Can you work these out from the model? Positions are in its coordinate system, mm. A direction names the side the tool comes from. Coordinates: 2 decimals unless noted, no trailing zeros. Write each loop counter-clockwise with the first axis right and the second up, starting at its lowest first coordinate (ties: lowest second). Pieces come first, ordered by that corner, then holes.
```python
from build123d import *

# Parameters (mm, degrees)
BOSS_EXTRUDE1_DEPTH  = 5
SKETCH8_W            = 12.7
SKETCH8_H            = 25.4
CUT_EXTRUDE1_DEPTH   = 12.7
BOSS_EXTRUDE6_START  = 1.27
BOSS_EXTRUDE6_DEPTH  = 22.86
FILLET3_R            = 2.54
SKETCH12_W           = 22.86
SKETCH12_H           = 5.08
BOSS_EXTRUDE7_DEPTH  = 5.08
FILLET8_R            = 2.54
SKETCH13_W           = 2.54
SKETCH13_H           = 17.78
CUT_EXTRUDE2_DEPTH   = 2.032
BOSS_EXTRUDE8_DEPTH  = 22.86
FILLET5_R            = 2.54
FILLET6_R            = 2.54
BOSS_EXTRUDE9_START  = -27.94
SKETCH15_W           = 10.16
SKETCH15_H           = 3.81
BOSS_EXTRUDE9_DEPTH  = 12.7
BOSS_EXTRUDE10_START = -116.84
SKETCH15_2_W         = 10.16
SKETCH15_2_H         = 3.81
BOSS_EXTRUDE10_DEPTH = 12.7
FILLET7_R            = 2.54


with BuildPart() as part:
    # Sketch2 → Boss-Extrude1 (new body)
    with BuildSketch(Plane(origin=(0, 0, 0), x_dir=(1, 0, 0), z_dir=(0, 1, 0))):
        with BuildLine():
            Line((-98.109845206, -87.510053172), (49.730154794, -87.510053172))
            ThreePointArc((49.730154794, -87.510053172), (53.322257243, -86.02215562), (54.810154794, -82.430053172))
            Line((54.810154794, -82.430053172), (54.810154794, 64.409946828))
            ThreePointArc((54.810154794, 64.409946828), (53.322257243, 68.002049277), (49.730154794, 69.489946828))
            Line((49.730154794, 69.489946828), (-98.109845206, 69.489946828))
            ThreePointArc((-98.109845206, 69.489946828), (-101.701947654, 68.002049277), (-103.189845206, 64.409946828))
            Line((-103.189845206, 64.409946828), (-103.189845206, -82.430053172))
            ThreePointArc((-103.189845206, -82.430053172), (-101.701947654, -86.02215562), (-98.109845206, -87.510053172))
        make_face()
    extrude(amount=BOSS_EXTRUDE1_DEPTH)

    # Sketch8 → Cut-Extrude1 (cut)
    with BuildSketch(Plane(origin=(0, 5, 0), x_dir=(1, 0, 0), z_dir=(0, 1, 0))):
        with Locations((-96.839845206, -9.250053172)):
            Rectangle(SKETCH8_W, SKETCH8_H)
    extrude(amount=-CUT_EXTRUDE1_DEPTH, mode=Mode.SUBTRACT)

    # Sketch9 → Boss-Extrude6 (add)
    with BuildSketch(Plane(origin=(0, 0, 21.950053172), x_dir=(-1, 0, 0), z_dir=(0, 0, -1)).offset(BOSS_EXTRUDE6_START)):
        with BuildLine():
            Line((90.489845206, 5), (90.489845206, -9.510091846))
            ThreePointArc((90.489845206, -9.510091846), (91.233793982, -11.30614307), (93.029845206, -12.050091846))
            Line((93.029845206, -12.050091846), (100.984663509, -12.050091846))
            ThreePointArc((100.984663509, -12.050091846), (102.780714734, -11.30614307), (103.524663509, -9.510091846))
            Line((103.524663509, -9.510091846), (103.524663509, 5))
            Line((103.524663509, 5), (100.984663509, 5))
            Line((100.984663509, 5), (100.984663509, -6.970091846))
            ThreePointArc((100.984663509, -6.970091846), (100.240714734, -8.76614307), (98.444663509, -9.510091846))
            Line((98.444663509, -9.510091846), (97.007254358, -9.510091846))
            add(Edge.make_bspline(
                [(93.029845206, -3.470974905), (93.181288834, -7.756398779), (97.007254358, -9.510091846)],
                knots=[0, 0, 0, 1, 1, 1], degree=2))
            Line((93.029845206, -3.470974905), (93.029845206, 5))
            Line((93.029845206, 5), (90.489845206, 5))
        make_face()
    extrude(amount=BOSS_EXTRUDE6_DEPTH)

    # Fillet3
    fillet3_edges = [part.edges().sort_by_distance(p)[0] for p in [
        (-90.489845206, 0, 9.250053172),
    ]]
    fillet(fillet3_edges, radius=FILLET3_R)

    # Sketch12 → Boss-Extrude7 (add)
    with BuildSketch(Plane.ZY.offset(103.524663509)):
        with Locations((9.250053172, 2.46)):
            Rectangle(SKETCH12_W, SKETCH12_H)
    extrude(amount=BOSS_EXTRUDE7_DEPTH)

    # Fillet8
    fillet8_edges = [part.edges().sort_by_distance(p)[0] for p in [
        (-100.984663509, 5, 9.250053172),
    ]]
    fillet(fillet8_edges, radius=FILLET8_R)

    # Sketch13 → Cut-Extrude2 (cut)
    with BuildSketch(Plane(origin=(0, 5, 0), x_dir=(1, 0, 0), z_dir=(0, 1, 0))):
        with Locations((-106.064663509, -9.250053172)):
            Rectangle(SKETCH13_W, SKETCH13_H)
    extrude(amount=-CUT_EXTRUDE2_DEPTH, mode=Mode.SUBTRACT)

    # Sketch14 → Boss-Extrude8 (add)
    with BuildSketch(Plane(origin=(0, 0, -2.179946828), x_dir=(-1, 0, 0), z_dir=(0, 0, -1))):
        Polygon((103.524663509, -4.576775108), (105.048663509, -4.576775108), (103.524663509, -7.370775108), align=None)
    extrude(amount=-BOSS_EXTRUDE8_DEPTH)

    # Fillet5
    fillet5_edges = [part.edges().sort_by_distance(p)[0] for p in [
        (-93.029845206, 5, 9.250053172),
    ]]
    fillet(fillet5_edges, radius=FILLET5_R)

    # Fillet6
    fillet6_edges = [part.edges().sort_by_distance(p)[0] for p in [
        (-108.604663509, -0.08, 9.250053172),
    ]]
    fillet(fillet6_edges, radius=FILLET6_R)

    # Sketch15 → Boss-Extrude9 (add)
    with BuildSketch(Plane(origin=(0, 0, -69.489946828), x_dir=(-1, 0, 0), z_dir=(0, 0, -1)).offset(BOSS_EXTRUDE9_START)):
        with Locations((-54.290154794, -1.905)):
            Rectangle(SKETCH15_W, SKETCH15_H)
    extrude(amount=-BOSS_EXTRUDE9_DEPTH)

    # Sketch15<2> → Boss-Extrude10 (add)
    with BuildSketch(Plane(origin=(0, 0, -69.489946828), x_dir=(-1, 0, 0), z_dir=(0, 0, -1)).offset(BOSS_EXTRUDE10_START)):
        with Locations((-54.290154794, -1.905)):
            Rectangle(SKETCH15_2_W, SKETCH15_2_H)
    extrude(amount=-BOSS_EXTRUDE10_DEPTH)

    # Fillet7
    # the kernel refuses this fillet: 2.54 mm, written as the material it adds along each edge
    with BuildSketch(Plane(origin=(49.210154794, 0, 47.350053172), x_dir=(-1, 0, 0), z_dir=(0, 0, 1)), Plane(origin=(49.210154794, 0, -41.549946828), x_dir=(-1, 0, 0), z_dir=(0, 0, 1))) as fillet7_piece_1:
        with BuildLine():
            CenterArc((FILLET7_R, FILLET7_R), FILLET7_R, 180, 90)
            Line((0, FILLET7_R), (0, 0))
            Line((0, 0), (FILLET7_R, 0))
        make_face()
    extrude(amount=12.7)
    # the kernel refuses this fillet: 2.54 mm, written as the material it takes off along each edge
    with BuildSketch(Plane(origin=(59.370154794, 0, 41.000053172), x_dir=(-1, 0, 0), z_dir=(0, 0, 1)), Plane(origin=(59.370154794, -3.81, 41.000053172), x_dir=(0, 1, 0), z_dir=(0, 0, 1)), Plane(origin=(59.370154794, -3.81, -47.899946828), x_dir=(0, 1, 0), z_dir=(0, 0, 1)), Plane(origin=(59.370154794, 0, -47.899946828), x_dir=(-1, 0, 0), z_dir=(0, 0, 1))) as fillet7_2_piece_1:
        with BuildLine():
            CenterArc((FILLET7_R, FILLET7_R), FILLET7_R, 180, 90)
            Line((0, FILLET7_R), (0, 0))
            Line((0, 0), (FILLET7_R, 0))
        make_face()
    extrude(amount=25.4, mode=Mode.SUBTRACT)


solid = part.part
```
1. If I drill on L1, parallel to X at y = -3.75, z = 11; L2, parallel to Y at x = -69, z = 59; L3, parallel to X at y = 1.75, z = 64, over which ranges is the centre line in solid material (lowest first)?
2. Which directions (+Z, -Z, +X, -X, +Y, -Y) give clear straight access to the entire face, cutting with the end or side of a thin tool? Please do faces 5 (the face through (54, -2, 47.35)), 6 (the face through (-103.19, 2, -34)), 7 (the face through (-93.03, -1, 9)), 8 (the face through (-103.525, -2, 9)), 9 (the face through (-97, 3, 21.95)).
3. If we section it at A-A, the plane z = 50: List the corners of the cut face in (x, y) for me (1 decimal), plus the area to 3 significant figures.
4. I'm going to push flat-ended pins straight in: P1, Ø0.6, axis at y = -3, z = -35.5, coming from the -X side; P2, Ø4, axis at x = -100, y = 2, coming from the +Z side; P3, Ø3, axis at y = -2, z = 15, coming from the -X side; P4, Ø4, axis at x = 54.5, z = 54.5, coming from the -Y side. Where does each tip first touch, or does it pass through?
5. If we section it at C-C, the plane z = 73.5: List the corners of the cut face in (x, y) for me.
6. We'd pull the mould along Z, two halves only. Please class faces 1 (the face through (-25, 5, 10)), 2 (the face through (54, -2, -41.55)), 3 (the face through (-100.985, -2, 9)), 4 (the face through (54, -2, 60.05)): released by +Z, released by -Z, zero draft, split by the parting line, or undercut.
7. If we section it at B-B, the plane x = -39.5: List the corners of the cut face in (y, z) for me, plus the area to 3 significant figures.
Answers:
1. L1: x = -103.52 to -100.98, -93.04 to -90.49
1. L2: y = 0 to 5
1. L3: x = -103.19 to 54.81
2. face 5: +X, -X, -Y
2. face 6: -Z, -X, +Y, -Y
2. face 7: +Y
2. face 8: +Z, -Z, -X
2. face 9: -X, +Y, -Y
3. outline: (-103.2, 0) - (46.7, 0) arc R2.5 cw to (49.2, -2.5) - (49.2, -3.8) - (56.8, -3.8) arc R2.5 ccw to (59.3, -1.9) arc R2.5 ccw to (56.8, 0) - (54.8, 0) - (54.8, 5) - (-103.2, 5) - close
3. area: 827 mm2
4. P1: stops at x = 49.21
4. P2: stops at z = 87.51
4. P3: stops at x = -103.52
4. P4: stops at y = -3.81
5. outline: (-103.19, 0) - (54.81, 0) - (54.81, 5) - (-103.19, 5) - close
6. face 1: zero draft
6. face 2: released by -Z
6. face 3: undercut
6. face 4: released by +Z
7. outline: (0, -69.49) - (5, -69.49) - (5, 87.51) - (0, 87.51) - close
7. area: 785 mm2
